from build123d import *

# Parameters (mm, degrees)
SKETCH1_R                = 13.5
BOSS_EXTRUDE1_DEPTH      = 18.5
BOSS_EXTRUDE2_DEPTH      = 3.5
BOSS_EXTRUDE2_DEPTH_BACK = 21.5
SKETCH3_R                = 1.5


with BuildPart() as part:
    # Sketch1 → Boss-Extrude1 (new body)
    with BuildSketch(Plane(origin=(0, 0, 0), x_dir=(1, 0, 0), z_dir=(0, 1, 0))):
        with Locations(Location((0, 0, 0), (0, 0, 270))):
            Circle(SKETCH1_R)
    extrude(amount=BOSS_EXTRUDE1_DEPTH)

    # Sketch2 → Cut-Revolve1 (revolve, cut)
    with BuildSketch(Plane.XY, mode=Mode.PRIVATE) as cut_revolve1_sk:
        Polygon((-13.5, 14), (-9, 18.5), (-13.5, 18.5), align=None)
    revolve(cut_revolve1_sk.sketch.rotate(Axis((0, 18.5, 0), (0, -1, 0)), 270), axis=Axis((0, 18.5, 0), (0, -1, 0)), mode=Mode.SUBTRACT)

    # Sketch3 → Boss-Extrude2 (add, two sides: drawn at the far end of the back side and taken through both)
    with BuildSketch(Plane(origin=(0, 18.5, 0), x_dir=(1, 0, 0), z_dir=(0, 1, 0)).offset(-BOSS_EXTRUDE2_DEPTH_BACK)):
        with Locations(Location((0, 0, 0), (0, 0, 270))):
            Circle(SKETCH3_R)
    extrude(amount=BOSS_EXTRUDE2_DEPTH + BOSS_EXTRUDE2_DEPTH_BACK)


solid = part.part
Can you work these out from the model? Positions are in its coordinate system, mm. A direction names the side the tool comes from. Give positions to 0.01 mm unless a question says otherwise; leave off trailing zeros. Order: outer loops, then holes, each group sorted by start corner. A loop starts at its lowest first (then second) coordinate and runs counter-clockwise, first axis right, second up. Notation, with made-up numbers: M 43,-1.5 L 93,-1.5 A11 cw 93,16.5 Z; hole C 79,47.25 d4. An arc over 180 degrees is marked long. Use a Markdown table: item, result. Add a question column.
Item 1: Suppose I cut it at D-D (y = 2.75). List the corners of the cut face in (x, z) for me.
Item 2: Suppose I cut it at B-B (z = 0). List the corners of the cut face in (x, y) for me, then the cut area to 3 significant figures.
Item 3: Suppose I cut it at A-A (x = 0). List the corners of the cut face in (y, z) for me, then the cut area to 3 significant figures.
Item 4: Will these pins go through, and if not, where does the flat tip stop? pin 1 (10 mm diameter, centred on x = 10.5, z = -6.5, fed in from -Y); pin 2 (8 mm diameter, centred on y = 18, z = -8, fed in from -X); pin 3 (4 mm diameter, centred on x = -10, z = 9.5, fed in from +Y).
Item 5: Suppose I cut it at C-C (y = 16). List the corners of the cut face in (x, z) for me.
Item 6: For faces 1 (the cylindrical face through (0.45, -1.52, 1.43)), 2 (the cylindrical face through (-13.18, 6.9, -2.93)), 3 (the cylindrical face through (0.45, 20.23, 1.43)), which set-ups out of +Z, -Z, +X, -X, +Y, -Y let a thin tool reach every point of the face, with its end or its side?
Item 7: If I drill on L1, parallel to Y at x = 0.25, z = -2; L2, parallel to Z at x = 3.75, y = 8.25; L3, parallel to X at y = 6.75, z = 12, over which ranges is the centre line in solid material (lowest first)? Write a range as [from, to].
Answer sheet:
| question | item | result |
|---|---|---|
| 1 | outline | C 0,0 d27 |
| 2 | outline | M -13.5,0 L -1.5,0 L -1.5,-3 L 1.5,-3 L 1.5,0 L 13.5,0 L 13.5,14 L 9,18.5 L 1.5,18.5 L 1.5,22 L -1.5,22 L -1.5,18.5 L -9,18.5 L -13.5,14 Z |
| 2 | area | 499 mm² |
| 3 | outline | M -3,-1.5 L 0,-1.5 L 0,-13.5 L 14,-13.5 L 18.5,-9 L 18.5,-1.5 L 22,-1.5 L 22,1.5 L 18.5,1.5 L 18.5,9 L 14,13.5 L 0,13.5 L 0,1.5 L -3,1.5 Z |
| 3 | area | 499 mm² |
| 4 | pin 1 | stops at y = 0 |
| 4 | pin 2 | stops at x = -11.51 |
| 4 | pin 3 | stops at y = 15.71 |
| 5 | outline | C 0,0 d23 |
| 6 | face 1 | -Y |
| 6 | face 2 | +Y, -Y |
| 6 | face 3 | +Y |
| 7 | L1 | y = [0, 18.5] |
| 7 | L2 | z = [-12.97, 12.97] |
| 7 | L3 | x = [-6.18, 6.18] |
